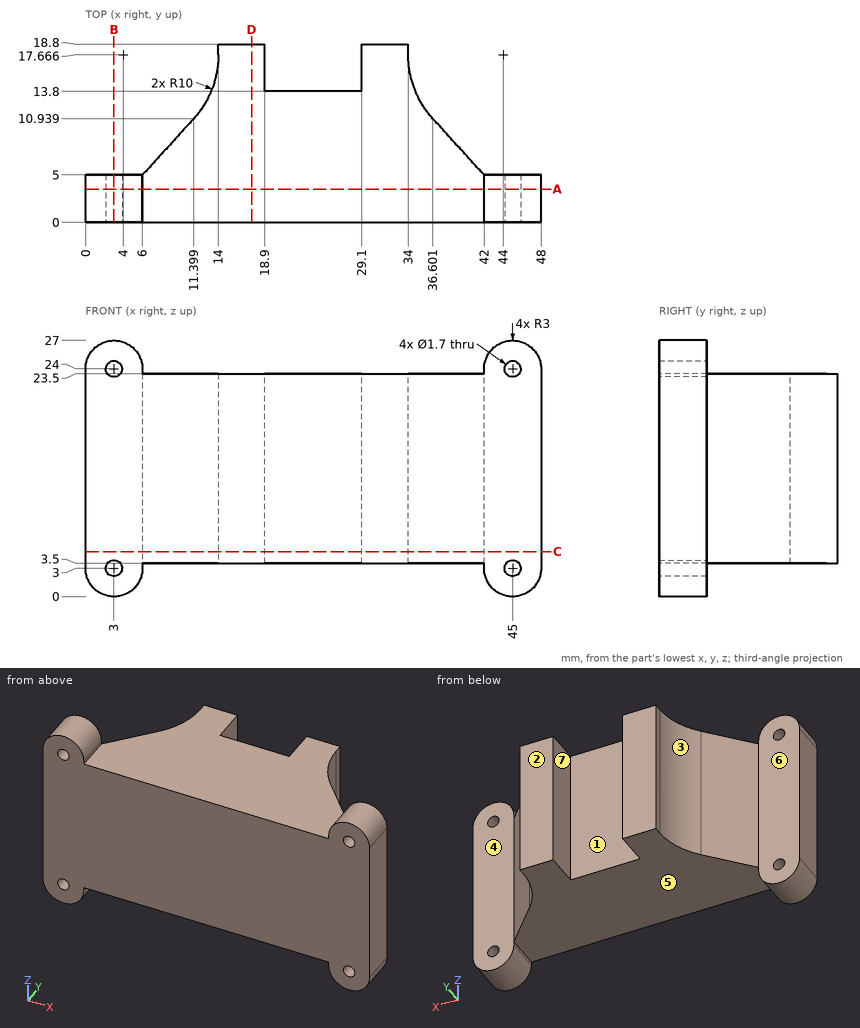
Answer from the drawing. Dimensions are ordinates in mm from the lowest x, y and z of the part. A direction names the side the tool comes from. Coordinates: 2 decimals unless noted, no trailing zeros. Write each loop counter-clockwise with the first axis right and the second up, starting at its lowest first coordinate (ties: lowest second). Pieces come first, ordered by that corner, then holes. Notation, with made-up numbers: M 17.25,-36.75 L 43.25,-36.75 A20 cw 43.25,-31.75 Z; hole C 42,-30 d1. An arc over 180 degrees is marked long. Use one line per item in the form item = value. Start each with the question number.
1. The part is cut by section B-B (x = 3). Give the vertices of the cut face in (y, z).
2. The part is cut by section D-D (x = 17.5). Give the vertices of the cut face in (y, z), plus the area to 3 significant figures.
3. The mould has two halves that part along X. Classify the marked faces 1, 2 and 3: released by +X, released by -X, zero draft, split by the parting line, or undercut.
4. A tool of negligible diameter and unlimited length cuts with its end or side. For the marked faces 4, 5, 6 and 7, from which of +Z, -Z, +X, -X, +Y, -Y can it reach the whole face along a straight path? Write none if from no direction.
5. Each of these flat-tipped pins is pushed along its axis until it touches: P1, Ø5, axis at y = 10, z = 19.5, coming from the -X side; P2, Ø2.5, axis at x = 3, z = 3, coming from the -Y side; P3, Ø2, axis at y = 14, z = 20.5, coming from the -X side (1 decimal); P4, Ø2.5, axis at y = 16, z = 11, coming from the -X side (1 decimal). Where does it stop, or does it pass through?
6. The part is cut by section A-A (y = 3.5). Give the vertices of the cut face in (x, z).
7. The part is cut by section C-C (z = 4.75). Give the vertices of the cut face in (x, y).
8. Straight lines are drawn through the part: probe 1 along Z at (x, y) = (45, 2.9); probe 2 along X at (y, z) = (3.75, 3); probe 3 along X at (y, z) = (17.75, 17). For each, find the intervals that lie inside material, in ascending order. Write a range as from..to.
Evaluation:
q1.outline = M 0,0 L 5,0 L 5,2.15 L 0,2.15 Z; M 0,3.85 L 5,3.85 L 5,23.15 L 0,23.15 Z; M 0,24.85 L 5,24.85 L 5,27 L 0,27 Z
q2.outline = M 0,3.5 L 18.8,3.5 L 18.8,23.5 L 0,23.5 Z
q2.area = 376 mm^2
q3.face_1 = undercut
q3.face_2 = zero draft
q3.face_3 = released by -X
q4.face_4 = +Z, -Z, +X, +Y
q4.face_5 = -Z, +Y, -Y
q4.face_6 = +Z, -Z, -X, +Y
q4.face_7 = +Z, -Z, +Y
q5.P1 = 8.27
q5.P2 = 0
q5.P3 = 12.8
q5.P4 = 13.6
q6.outline = M 0,3 A3 ccw 6,3 L 6,3.5 L 42,3.5 L 42,3 A3 ccw 48,3 L 48,24 A3 ccw 42,24 L 42,23.5 L 6,23.5 L 6,24 A3 ccw 0,24 Z; hole C 3,3 d1.7; hole C 3,24 d1.7; hole C 45,3 d1.7; hole C 45,24 d1.7
q7.outline = M 0,0 L 48,0 L 48,5 L 42,5 L 36.6,10.94 A10 cw 34,17.67 L 34,18.8 L 29.1,18.8 L 29.1,13.8 L 18.9,13.8 L 18.9,18.8 L 14,18.8 L 14,17.67 A10 cw 11.4,10.94 L 6,5 L 0,5 Z
q8.probe_1 = 0..2.15, 3.85..23.15, 24.85..27
q8.probe_2 = 0..2.15, 3.85..6, 42..44.15, 45.85..48
q8.probe_3 = 14..18.9, 29.1..34
